```python
from build123d import *
from build123d.topology import SkipClean

# Parameters (mm, degrees)
SKETCH_1_R           = 31.5
EXTRUDE_1_DEPTH      = 60
SKETCH_4_W           = 221.5
SKETCH_4_H           = 50
EXTRUDE_2_DEPTH      = 50
SKETCH_5_W           = 2.75
SKETCH_5_H           = 15
CUT_EXTRUDE_1_DEPTH  = 126.530125866
SKETCH_6_R           = 17
EXTRUDE_3_DEPTH      = 3
SKETCH_7_R           = 10
CUT_EXTRUDE_2_DEPTH  = 45
SKETCH_8_R           = 1.5
CUT_EXTRUDE_3_DEPTH  = 127.340066883
EXTRUDE_4_DEPTH      = 3
SKETCH_10_R          = 3.25
CUT_EXTRUDE_4_DEPTH  = 127.754930871
CUT_EXTRUDE_5_DEPTH  = 121.344557417
SKETCH_12_R          = 24
EXTRUDE_5_DEPTH      = 17
SKETCH_13_W          = 48
SKETCH_13_H          = 23
EXTRUDE_6_DEPTH      = 28
CUT_EXTRUDE_6_DEPTH  = 131.65053582
FILLET_1_R           = 12
CUT_EXTRUDE_7_DEPTH  = 8
SKETCH_17_R          = 9
CUT_EXTRUDE_8_DEPTH  = 13
SKETCH_18_R          = 5.5
CUT_EXTRUDE_9_DEPTH  = 144.968963711
SKETCH_19_R          = 20
CUT_EXTRUDE_10_DEPTH = 135.794519592
SKETCH_20_W          = 2
SKETCH_20_H          = 52.086738744
CUT_EXTRUDE_11_DEPTH = 135.794519592
M6X1_0_1_AT_2_COUNT  = 2
M6X1_0_1_AT_2_PITCH  = 35
M6X1_0_1_AT_3_COUNT  = 2
M6X1_0_1_AT_3_PITCH  = 49.500749042
M6X1_0_1_AT_4_COUNT  = 2
M6X1_0_1_AT_4_PITCH  = 35
FILLET_2_R           = 2


with BuildPart() as part:
    # 草图1 → 凸台-拉伸1 (new body)
    with BuildSketch(Plane.XY):
        Circle(SKETCH_1_R)
    extrude(amount=EXTRUDE_1_DEPTH)

    # 草图4 → 凸台-拉伸2 (add)
    with BuildSketch(Plane.XY):
        Rectangle(SKETCH_4_W, SKETCH_4_H)
    extrude(amount=EXTRUDE_2_DEPTH)

    # 草图5 → 切除-拉伸1 (cut, through all)
    with BuildSketch(Plane.XY.offset(50)):
        with Locations((-109.375, 17.5)):
            Rectangle(SKETCH_5_W, SKETCH_5_H)
        with Locations((-109.375, -17.5)):
            Rectangle(SKETCH_5_W, SKETCH_5_H)
        with Locations((109.375, -17.5)):
            Rectangle(SKETCH_5_W, SKETCH_5_H)
        with Locations((109.375, 17.5)):
            Rectangle(SKETCH_5_W, SKETCH_5_H)
    extrude(amount=-CUT_EXTRUDE_1_DEPTH, mode=Mode.SUBTRACT)

    # 草图6 → 凸台-拉伸3 (add)
    with BuildSketch(Plane.XY.offset(50)):
        with Locations((-80, 0)):
            Circle(SKETCH_6_R)
        with Locations(Location((80, 0, 0), (0, 0, 180))):
            Circle(SKETCH_6_R)
    extrude(amount=EXTRUDE_3_DEPTH)

    # 草图7 → 切除-拉伸2 (cut)
    with BuildSketch(Plane.XY.offset(53)):
        with Locations((-80, 0)):
            Circle(SKETCH_7_R)
        with Locations((80, 0)):
            Circle(SKETCH_7_R)
    extrude(amount=-CUT_EXTRUDE_2_DEPTH, mode=Mode.SUBTRACT)

    # 草图8 → 切除-拉伸3 (cut, through all)
    with BuildSketch(Plane.XY.offset(8)):
        with Locations((-80, 0)):
            Circle(SKETCH_8_R)
        with Locations((80, 0)):
            Circle(SKETCH_8_R)
    extrude(amount=-CUT_EXTRUDE_3_DEPTH, mode=Mode.SUBTRACT)

    # 草图9 → 凸台-拉伸4 (add)
    with BuildSketch(Plane.XY.offset(50)):
        with BuildLine():
            Line((-30.467195473, 8), (-45, 8))
            ThreePointArc((-45, 8), (-53, 0), (-45, -8))
            Line((-45, -8), (-30.467195473, -8))
            ThreePointArc((-30.467195473, -8), (-31.5, 0), (-30.467195473, 8))
        make_face()
    extrude(amount=EXTRUDE_4_DEPTH)

    # 草图10 → 切除-拉伸4 (cut, through all)
    with BuildSketch(Plane.XY.offset(53)):
        with Locations((-45, 0)):
            Circle(SKETCH_10_R)
    extrude(amount=-CUT_EXTRUDE_4_DEPTH, mode=Mode.SUBTRACT)

    # 草图11 → 切除-拉伸5 (cut, through all)
    with SkipClean():  # the faces are left unmerged after this step: merging them gives an invalid solid
        with BuildSketch(Plane.XY.offset(35)):
            with BuildLine():
                Line((-59.287684823, 14), (-28.217902119, 14))
                ThreePointArc((-28.217902119, 14), (-24.320889444, 20.018599767), (-19.163767897, 25))
                Line((-19.163767897, 25), (-80, 25))
                ThreePointArc((-80, 25), (-68.2739606, 22.079402166), (-59.287684823, 14))
            make_face()
            with BuildLine():
                Line((80, 25), (19.163767897, 25))
                ThreePointArc((19.163767897, 25), (24.320889444, 20.018599767), (28.217902119, 14))
                Line((28.217902119, 14), (59.287684823, 14))
                ThreePointArc((59.287684823, 14), (68.2739606, 22.079402166), (80, 25))
            make_face()
        cut_extrude_5 = extrude(amount=CUT_EXTRUDE_5_DEPTH, mode=Mode.SUBTRACT)

    # 镜向1: 切除-拉伸5 across plane
    with SkipClean():  # the faces are left unmerged after this step: merging them gives an invalid solid
        add(cut_extrude_5.mirror(Plane(origin=(0, 0, 25), x_dir=(1, 0, 0), z_dir=(0, 0, -1))), mode=Mode.SUBTRACT)
    add(part.part.scale(1), mode=Mode.REPLACE)  # the faces are merged on a copy

    # 草图12 → 凸台-拉伸5 (add)
    with BuildSketch(Plane(origin=(0, 25, 0), x_dir=(1, 0, 0), z_dir=(0, 1, 0))):
        with Locations(Location((0, -25, 0), (0, 0, 37.013819742))):
            Circle(SKETCH_12_R)
    extrude(amount=EXTRUDE_5_DEPTH)

    # 草图13 → 凸台-拉伸6 (add)
    with BuildSketch(Plane(origin=(0, 0, 18), x_dir=(-1, 0, 0), z_dir=(0, 0, -1))):
        with Locations((0, -36.5)):
            Rectangle(SKETCH_13_W, SKETCH_13_H)
    extrude(amount=-EXTRUDE_6_DEPTH)

    # 草图14 → 切除-拉伸6 (cut, through all)
    with BuildSketch(Plane.XY.offset(50)):
        with BuildLine():
            Line((-80, -25), (-24, -25))
            Line((-24, -25), (-28.217902119, -14))
            Line((-28.217902119, -14), (-59.287684823, -14))
            ThreePointArc((-59.287684823, -14), (-68.2739606, -22.079402166), (-80, -25))
        make_face()
        with BuildLine():
            Line((28.217902119, -14), (24, -25))
            Line((24, -25), (80, -25))
            ThreePointArc((80, -25), (68.2739606, -22.079402166), (59.287684823, -14))
            Line((59.287684823, -14), (28.217902119, -14))
        make_face()
    extrude(amount=-CUT_EXTRUDE_6_DEPTH, mode=Mode.SUBTRACT)

    # 圆角1
    # the kernel refuses this fillet: 12 mm, written as the material it adds along each edge
    with BuildSketch(Plane(origin=(-28.217902119, -14, 50), x_dir=(0.3580274430169819, -0.9337110634702374, 0), z_dir=(0, 0, -1)), Plane(origin=(28.217902119, -14, 50), x_dir=(1, 0, 0), z_dir=(0, 0, -1))) as fillet_1_piece_1:
        with BuildLine():
            CenterArc((FILLET_1_R * 0.687549480882, FILLET_1_R), FILLET_1_R, 200.979103866, 69.020896134)
            Line((-FILLET_1_R * 0.246161582588, FILLET_1_R * 0.641972556983), (0, 0))
            Line((0, 0), (FILLET_1_R * 0.687549480882, 0))
        make_face()
    extrude(amount=50)

    # 草图15 → 切除-拉伸7 (cut)
    with BuildSketch(Plane.ZY.offset(24)):
        Polygon((32, -24.607695155), (23, -29.803847577), (23, -40.196152423), (32, -45.392304845), (41, -40.196152423), (41, -29.803847577), align=None)
    extrude(amount=-CUT_EXTRUDE_7_DEPTH, mode=Mode.SUBTRACT)

    # 草图17 → 切除-拉伸8 (cut)
    with BuildSketch(Plane(origin=(24, 0, 0), x_dir=(0, 0, -1), z_dir=(1, 0, 0))):
        with Locations(Location((-32, -35, 0), (0, 0, 90))):
            Circle(SKETCH_17_R)
    extrude(amount=-CUT_EXTRUDE_8_DEPTH, mode=Mode.SUBTRACT)

    # 草图18 → 切除-拉伸9 (cut, through all)
    with BuildSketch(Plane(origin=(11, 0, 0), x_dir=(0, 0, -1), z_dir=(1, 0, 0))):
        with Locations(Location((-32, -35, 0), (0, 0, 90))):
            Circle(SKETCH_18_R)
    extrude(amount=-CUT_EXTRUDE_9_DEPTH, mode=Mode.SUBTRACT)

    # 草图19 → 切除-拉伸10 (cut, through all)
    with BuildSketch(Plane.XY.offset(60)):
        Circle(SKETCH_19_R)
    extrude(amount=-CUT_EXTRUDE_10_DEPTH, mode=Mode.SUBTRACT)

    # 草图20 → 切除-拉伸11 (cut, through all)
    with BuildSketch(Plane.XY.offset(60)):
        with Locations((0, -32.440330594)):
            Rectangle(SKETCH_20_W, SKETCH_20_H)
    extrude(amount=-CUT_EXTRUDE_11_DEPTH, mode=Mode.SUBTRACT)

    # 草图21 → M6x1.0 螺纹孔1 (revolve, cut)
    with BuildSketch(Plane(origin=(-108, 17.505623263, 42.5), x_dir=(0, 0, 1), z_dir=(0, 1, 0))):
        Polygon((0, 0), (0, 16.502151548), (2.5, 15), (2.5, 0), align=None)
    m6x1_0_1 = revolve(axis=Axis((-114.35, 17.505623263, 42.5), (1, 0, 0)), mode=Mode.SUBTRACT)

    # M6x1.0 螺纹孔1 at 2: M6x1.0 螺纹孔1 ×2
    with Locations(*[(0, 0, -i * M6X1_0_1_AT_2_PITCH) for i in range(1, M6X1_0_1_AT_2_COUNT)]):
        add(m6x1_0_1, mode=Mode.SUBTRACT)

    # M6x1.0 螺纹孔1 at 3: M6x1.0 螺纹孔1 ×2
    with Locations(*[Vector(0, -0.7072471015902798, -0.7069664329316834) * (i * M6X1_0_1_AT_3_PITCH) for i in range(1, M6X1_0_1_AT_3_COUNT)]):
        add(m6x1_0_1, mode=Mode.SUBTRACT)

    # M6x1.0 螺纹孔1 at 4: M6x1.0 螺纹孔1 ×2
    with Locations(*[Vector(0, -0.9999999912472337, 0.0001323084749892749) * (i * M6X1_0_1_AT_4_PITCH) for i in range(1, M6X1_0_1_AT_4_COUNT)]):
        add(m6x1_0_1, mode=Mode.SUBTRACT)

    # 镜向2: M6x1.0 螺纹孔1 across plane
    add(m6x1_0_1.mirror(Plane(origin=(0, 0, 0), x_dir=(0, 0, 1), z_dir=(1, 0, 0))), mode=Mode.SUBTRACT)

    # 镜向2 copy 1 sketch → 镜向2 copy 1 (revolve, cut)
    with BuildSketch(Plane(origin=(108, 17.505623263, 7.5), x_dir=(0, 0, 1), z_dir=(0, 1, 0))):
        Polygon((0, 0), (0, -16.502151548), (2.5, -15), (2.5, 0), align=None)
    revolve(axis=Axis((114.35, 17.505623263, 7.5), (1, 0, 0)), mode=Mode.SUBTRACT)

    # 镜向2 copy 2 sketch → 镜向2 copy 2 (revolve, cut)
    with BuildSketch(Plane(origin=(108, -17.503638023, 7.504632022), x_dir=(0, 0, 1), z_dir=(0, 1, 0))):
        Polygon((0, 0), (0, -16.502151548), (2.5, -15), (2.5, 0), align=None)
    revolve(axis=Axis((114.35, -17.503638023, 7.504632022), (1, 0, 0)), mode=Mode.SUBTRACT)

    # 镜向2 copy 3 sketch → 镜向2 copy 3 (revolve, cut)
    with BuildSketch(Plane(origin=(108, -17.49437643, 42.504630797), x_dir=(0, 0, 1), z_dir=(0, 1, 0))):
        Polygon((0, 0), (0, -16.502151548), (2.5, -15), (2.5, 0), align=None)
    revolve(axis=Axis((114.35, -17.49437643, 42.504630797), (1, 0, 0)), mode=Mode.SUBTRACT)

    # 圆角2
    fillet_2_edges = [part.edges().sort_by_distance(p)[0] for p in [
        (28.217902119, 14, 42.5),
        (-59.287684823, 14, 42.5),
        (28.217902119, 14, 7.5),
        (-59.287684823, 14, 7.5),
    ]]
    fillet(fillet_2_edges, radius=FILLET_2_R)


solid = part.part
```
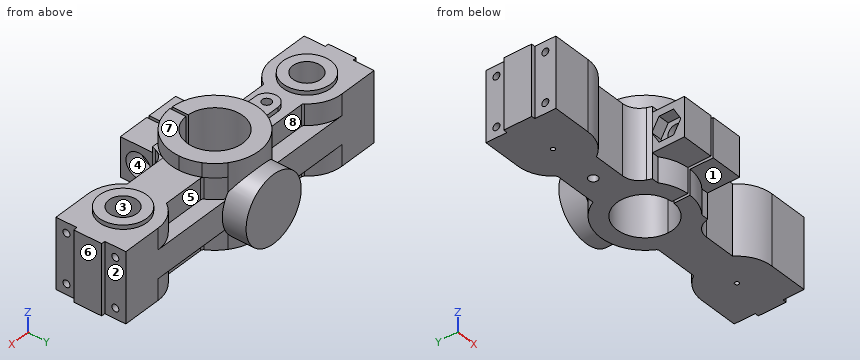
Part model, mm, in its own coordinate system. Face numbers are marked on the shaded views. A direction names the side the tool comes from. Coordinates: 2 decimals unless noted, no trailing zeros. Order: outer loops, then holes, each group sorted by start corner. A loop starts at its lowest first (then second) coordinate and runs counter-clockwise, first axis right, second up. Notation, with made-up numbers: (-32, -10.75) - (-13, -10.75) arc R24 ccw to (-13, 9.25) - close; hole circle Ø1 at (15.5, -3.5). An arc over 180 degrees is marked (long way). Return JSON: item names as keys, results as strings. Group by question number.
Item 1: Pull direction X, two halves, no side cores. Call the marked faces 6, 7 and 8: pulls with the +X half, pulls with the -X half, needs draft (parallel to the pull), parting line crosses it, or undercut.
Item 2: Drill centre lines: probe 1 along X at (y, z) = (0.5, 17); probe 2 along Y at (x, z) = (97.25, 7.5); probe 3 along X at (y, z) = (-39, 38). Where is each one in solid material? Low to high. Write a range as from..to.
Item 3: Cut at A-A (x = 45.5). List the corners of the cut face in (y, z).
Item 4: Which spindle directions (+Z, -Z, +X, -X, +Y, -Y) get a long thin tool onto all of the face, cutting with end or side? Do the marked faces 1, 2, 3, 4 and 5. Say none if no direction does.
Item 5: Cut at B-B (z = 55). List the corners of the cut face in (x, y), plus the area to 3 significant figures.
Item 6: Pin check, flat tips, straight feed: pin 1 (3.5 mm diameter, centred on x = 80, y = 0, fed in from +Z); pin 2 (3 mm diameter, centred on x = -108.5, z = 12.5, fed in from +Y); pin 3 (22.5 mm diameter, centred on y = -30, z = 43.5, fed in from +X). Stop position of each tip, or through.
Check values:
{
 "1": {"face 6": "pulls with the +X half", "face 7": "needs draft", "face 8": "undercut"},
 "2": {"probe 1": "x = -110.75..-89.99, -70.01..-48.21, -41.79..-19.99, 19.99..70.01, 89.99..110.75", "probe 2": "y = -25..-20, -15..15.01, 20.01..25", "probe 3": "x = -16..-1, 1..11"},
 "3": {"outline": "(-14, 0) - (14, 0) - (14, 15) - (25, 15) - (25, 35) - (14, 35) - (14, 50) - (-14, 50) - close"},
 "4": {"face 1": "-Z, +X, -Y", "face 2": "+Z, -Z, +X, +Y", "face 3": "+Z", "face 4": "+X", "face 5": "+Z, +Y"},
 "5": {"outline": "(-1, -31.48) - (-1, -19.97) arc R20 cw (long way) to (1, -19.97) - (1, -31.48) arc R31.5 ccw (long way) to start", "area": "1,840 mm2"},
 "6": {"pin 1": "stops at z = 8", "pin 2": "stops at y = 25", "pin 3": "stops at x = 108"}
}
